Work out the finished part from the listing and answer in its coordinate system (mm). A direction names the side the tool comes from. Round coordinates to 2 decimals unless told otherwise and drop trailing zeros. Order: outer loops, then holes, each group sorted by start corner. A loop starts at its lowest first (then second) coordinate and runs counter-clockwise, first axis right, second up. Notation, with made-up numbers: (48.25, 0) -> (99.25, 0) arc R28 cw to (99.25, 20) -> close; hole circle Ø6 at (15.5, 55). An arc over 180 degrees is marked (long way). Use a Markdown table: item, result. Add a question column.
Item 1: A cutting plane is placed at D-D, the plane x = 5.75. Determine the outline of the cut face in (y, z) (3 decimals).
Item 2: A tool of negligible diameter and unlimited length cuts with its end or side. For faces 4 (the cylindrical face through (9.436, 4.346, -2.26)), 5 (the flat face through (0, 3.2, 1)), 6 (the cylindrical face through (16.76, 4.65, 1.03)), from which of +Z, -Z, +X, -X, +Y, -Y can it reach the whole face along a straight path? Write none if from no direction.
Item 3: Flat-ended cylindrical pins translate along their axes: P1, Ø3, axis at x = 3, z = 4, coming from the -Y side; P2, Ø2, axis at y = 4, z = 0.5, coming from the -X side; P3, Ø1.5, axis at x = 6.5, z = 4, coming from the -Y side; P4, Ø1.5, axis at x = 12, z = -2, coming from the -Y side. Find the tip coordinate at first contact, or state that the pin passes through.
Item 4: For a pull along Y with two mould halves and no side action, classify faces 1 (the cylindrical face through (9.13, -3.1, 0.69)), 2 (the flat face through (15.471, -5, -1)), 3 (the cylindrical face through (13.86, 3.86, 5.04)) as +Y half, -Y half, draft (parallel to the pull), parting line (faces both ways), or undercut.
Item 5: Find the intervals of material crossed by L1, parallel to Y at x = 13, z = 0 (3 decimals); L2, parallel to Y at x = 8.75, z = 0 (3 decimals); L3, parallel to Z at x = 6, y = 1, in increasing order. Write a range as [from, to].
from build123d import *

# Parameters (mm, degrees)
F_1_4_0_25_DIAMETER_HOLE1_D = 6.35


with BuildPart() as part:
    # Sketch1 → Revolve1 (revolve)
    with BuildSketch(Plane.XY, mode=Mode.PRIVATE) as revolve1_sk:
        with BuildLine():
            Line((0, 0), (0, 4.89857161))
            ThreePointArc((0, 4.89857161), (4.040605918, 6.35), (8.081211835, 4.89857161))
            Line((8.081211835, 4.89857161), (10.753463242, 4.89857161))
            Line((10.753463242, 4.89857161), (12.204891632, 6.35))
            Line((12.204891632, 6.35), (15.470605918, 6.35))
            Line((15.470605918, 6.35), (15.470605918, 4.7625))
            Line((15.470605918, 4.7625), (18.010605918, 4.7625))
            Line((18.010605918, 4.7625), (18.010605918, 0))
            Line((18.010605918, 0), (0, 0))
        make_face()
    revolve(revolve1_sk.sketch.rotate(Axis((18.010605918, 0, 0), (-1, 0, 0)), 90), axis=Axis((18.010605918, 0, 0), (-1, 0, 0)))

    # 1_4 _0.25_ Diameter Hole1 (through all)
    with Locations(Plane.ZY):
        with Locations((0, 0)):
            Hole(F_1_4_0_25_DIAMETER_HOLE1_D / 2)


solid = part.part
Reported:
| question | item | result |
|---|---|---|
| 1 | outline | circle Ø12.231 at (0, 0); hole circle Ø6.35 at (0, 0) |
| 2 | face 4 | none |
| 2 | face 5 | +Z, -Z, -X, +Y, -Y |
| 2 | face 6 | +X |
| 3 | P1 | y = -5.78 |
| 3 | P2 | x = 0 |
| 3 | P3 | y = -4.98 |
| 3 | P4 | y = -6.22 |
| 4 | face 1 | undercut |
| 4 | face 2 | draft |
| 4 | face 3 | parting line |
| 5 | L1 | [-6.35, -3.175], [3.175, 6.35] |
| 5 | L2 | [-4.899, -3.175], [3.175, 4.899] |
| 5 | L3 | [-5.96, -3.01], [3.01, 5.96] |
